Read the model definition and answer for the solid it produces. Units are mm, in the model's axes. A direction names the side the tool comes from. Give positions to 0.01 mm unless a question says otherwise; leave off trailing zeros. Loops run counter-clockwise (first coordinate to the right, second up) from the corner with the lowest first, then second, coordinate; pieces in that order, holes last. Notation, with made-up numbers: M 35.25,5 L 42.25,5 A20 cw 42.25,38 Z; hole C 43,44.5 d5. An arc over 180 degrees is marked long. Return JSON: item names as keys, results as strings. Group by question number.
Autodesk Inventor part; units mm, degrees
ref_plane "YZ Plane" through (0, 0, 0) normal (1, 0, 0) x (0, 1, 0)
ref_plane "XZ Plane" through (0, 0, 0) normal (0, 1, 0) x (-1, 0, 0)
ref_plane "XY Plane" through (0, 0, 0) normal (0, 0, 1) x (1, 0, 0)
sketch "スケッチ1" plane through (0, 0, 0) normal (0, 0, 1) x (1, 0, 0)
  line L0 (7.5, 15) -> (-7.5, 15)
  line L1 (-7.5, 15) -> (-7.5, -15)
  line L2 (-7.5, -15) -> (7.5, -15)
  line L3 (7.5, -15) -> (7.5, 15)
  line L4 (7.5, 15) -> (-7.5, -15) construction
  line L5 (-7.5, 15) -> (7.5, -15) construction
  line L6 (-5.5, 13) -> (5.5, 13)
  line L7 (5.5, 13) -> (5.5, -13)
  line L8 (5.5, -13) -> (-5.5, -13)
  line L9 (-5.5, -13) -> (-5.5, 13)
  point P0 (0, 0)
  dimension "d0" = 15
  dimension "d1" = 30
  dimension "d2" = 2
extrude "押し出し1" add sketch "スケッチ1" along normal blind 280
sketch "スケッチ2" plane through (-7.5, 15, 0) normal (0, 1, 0) x (1, 0, 0)
  circle A0 centre (7.5, -10) radius 1.6
  circle A1 centre (7.5, -25) radius 1.6
  circle A2 centre (7.5, -40) radius 1.6
  line L0 (15, 0) -> (0, 0)
  circle A3 centre (7.5, -270) radius 1.6
  circle A4 centre (7.5, -255) radius 1.6
  line L1 (15, -280) -> (0, -280)
  point P0 (7.5, 0)
  point P1 (7.5, 0)
  dimension "d5" = 3.2
  dimension "d6" = 3.2
  dimension "d7" = 3.2
  dimension "d8" = 10
  dimension "d9" = 15
  dimension "d10" = 15
  dimension "d11" = 3.2
  dimension "d12" = 3.2
  dimension "d13" = 10
  dimension "d14" = 15
extrude "押し出し2" cut sketch "スケッチ2" against normal through all
properties part number "オムニ_角柱2" material "アルミニウム 6061"
1. Flat-ended cylindrical pins translate along their axes: P1, Ø3.5, axis at x = 0, z = 25, coming from the -Y side; P2, Ø2.5, axis at x = 0, z = 255, coming from the +Y side. Find the tip coordinate at first contact, or state that the pin passes through.
2. Find section A-A (y = -4.5). Write down the section's boundary in (x, z).
3. For faces 5 (the flat face through (0, -13, 138)), 6 (the flat face through (-7.5, 0, 138)), determine the directions among +Z, -Z, +X, -X, +Y, -Y from which every point of the face is accessible in a straight line to the end or side of a thin tool.
4. Straight lines are drawn through the part: line 1 along Z through (x, y) = (0, -13.4); line 2 along Y through (x, z) = (-5, 43); line 3 along X through (y, z) = (-7, 259.5). For each, find the intervals that lie inside material, in ascending order.
5. The mould has two halves that part along Y. Classify faces 1 (the flat face through (7.5, 0, 138)), 2 (the flat face through (-5.5, 0, 138)), 3 (the flat face through (0, -15, 138)), 4 (the flat face through (0, 13, 138)): +Y half, -Y half, draft (parallel to the pull), parting line (faces both ways), or undercut.
6. Find section B-B (z = 248). Write down the section's boundary in (x, y), and give its area (3 significant figures).
Result:
{
 "1": {"P1": "stops at y = -15", "P2": "passes through"},
 "2": {"outline": "M -7.5,0 L -5.5,0 L -5.5,280 L -7.5,280 Z; M 5.5,0 L 7.5,0 L 7.5,280 L 5.5,280 Z"},
 "3": {"face 5": "+Z, -Z", "face 6": "+Z, -Z, -X, +Y, -Y"},
 "4": {"line 1": "z = 0 to 8.4, 11.6 to 23.4, 26.6 to 38.4, 41.6 to 253.4, 256.6 to 268.4, 271.6 to 280", "line 2": "y = -15 to -13, 13 to 15", "line 3": "x = -7.5 to -5.5, 5.5 to 7.5"},
 "5": {"face 1": "draft", "face 2": "undercut", "face 3": "-Y half", "face 4": "undercut"},
 "6": {"outline": "M -7.5,-15 L 7.5,-15 L 7.5,15 L -7.5,15 Z; hole M -5.5,-13 L 5.5,-13 L 5.5,13 L -5.5,13 Z", "area": "164 mm2"}
}
